Read the model definition and answer for the solid it produces. Units are mm, in the model's axes. Round coordinates to 2 decimals unless told otherwise and drop trailing zeros. Write each loop counter-clockwise with the first axis right and the second up, starting at its lowest first coordinate (ties: lowest second). Pieces come first, ordered by that corner, then holes. Notation, with made-up numbers: M 25.25,29.25 L 49.25,29.25 A30 cw 49.25,63.25 Z; hole C 2,-39.75 d3. An arc over 180 degrees is marked long. Use one line per item in the form item = value. Start each with the question number.
```python
from build123d import *

# Parameters (mm, degrees)
SKETCH1_R               = 4.78
BOSS_EXTRUDE1_DEPTH     = 9.78
CUT_EXTRUDE1_DEPTH      = 12.888868743
CUT_EXTRUDE1_DEPTH_BACK = 12.888868743
SKETCH3_R               = 3.34
CHAMFER1_SIZE           = 0.76


with BuildPart() as part:
    # Sketch1 → Boss-Extrude1 (new, symmetric)
    with BuildSketch(Plane(origin=(0, 0, 0), x_dir=(0, 0, -1), z_dir=(1, 0, 0))):
        Circle(SKETCH1_R)
    extrude(amount=BOSS_EXTRUDE1_DEPTH, both=True)

    # Sketch3 → Cut-Extrude1 (cut, two sides: drawn at the far end of the back side and taken through both)
    with BuildSketch(Plane.XY.offset(-CUT_EXTRUDE1_DEPTH_BACK)):
        with Locations(Location((0, -0.25, 0), (0, 0, 4.292620915))):
            Circle(SKETCH3_R)
    extrude(amount=CUT_EXTRUDE1_DEPTH + CUT_EXTRUDE1_DEPTH_BACK, mode=Mode.SUBTRACT)

    # Chamfer1
    chamfer1_edges = [part.edges().sort_by_distance(p)[0] for p in [
        (-9.78, 0, 4.78),
        (9.78, 0, 4.78),
    ]]
    chamfer(chamfer1_edges, length=CHAMFER1_SIZE)


solid = part.part
```
Q1. Find section C-C on x = 0. Write down the section's boundary in (y, z), and give its area (3 significant figures).
Q2. Find section A-A on y = 0. Write down the section's boundary in (x, z), and give its area (3 significant figures).
Q3. Find section D-D on x = 6.5. Write down the section's boundary in (y, z).
Q4. Find section B-B on z = 0. Write down the section's boundary in (x, y), and give its area (3 significant figures).
Q5. Each of these flat-tipped pins is pushed along its axis until it touches: pin 1 Ø1.5 at (x, y) = (1.5, -2.5) entering from +Z; pin 2 Ø1.5 at (x, z) = (-5, 3.5) entering from -Y; pin 3 Ø1 at (y, z) = (-3, -3.5) entering from +X. Where does it stop, or does it pass through?
Q6. For a pull along Y with two mould halves and no side action, classify faces 1 (the face through (0.13, 4.74, 0.62)), 2 (the face through (-0.68, 3.02, -0.07)), 3 (the face through (9.78, 0, 0)) as +Y half, -Y half, draft (parallel to the pull), parting line (faces both ways), or undercut.
Q7. Straight lines are drawn through the part: line 1 (X direction, y = -0.25, z = 1); line 2 (Y direction, x = 0, z = -2); line 3 (Y direction, x = 0, z = 2.5). For each, find the intervals that lie inside material, in ascending order. Write a range as [from, to].
Response:
q1.outline = M -3.59,-3.16 L -3.59,3.16 A4.78 ccw Z; M 3.09,-3.65 A4.78 ccw 3.09,3.65 Z
q1.area = 13.7 mm²
q2.outline = M -9.78,-4.02 L -9.02,-4.78 L -3.33,-4.78 L -3.33,4.78 L -9.02,4.78 L -9.78,4.02 Z; M 3.33,-4.78 L 9.02,-4.78 L 9.78,-4.02 L 9.78,4.02 L 9.02,4.78 L 3.33,4.78 Z
q2.area = 122 mm²
q3.outline = C 0,0 d9.56
q4.outline = M -9.78,-4.02 L -9.02,-4.78 L 9.02,-4.78 L 9.78,-4.02 L 9.78,4.02 L 9.02,4.78 L -9.02,4.78 L -9.78,4.02 Z; hole C 0,-0.25 d6.68
q4.area = 151 mm²
q5.pin_1 = 3.9
q5.pin_2 = -3.91
q5.pin_3 = 9.69
q6.face_1 = parting line
q6.face_2 = undercut
q6.face_3 = draft
q7.line_1 = [-9.78, -3.34], [3.34, 9.78]
q7.line_2 = [-4.34, -3.59], [3.09, 4.34]
q7.line_3 = [-4.07, -3.59], [3.09, 4.07]
